Read the model definition and answer for the solid it produces. Units are mm, in the model's axes. Face numbers are marked on the shaded views. A direction names the side the tool comes from. Give positions to 0.01 mm unless a question says otherwise; leave off trailing zeros. Loops run counter-clockwise (first coordinate to the right, second up) from the corner with the lowest first, then second, coordinate; pieces in that order, holes last. Notation, with made-up numbers: (34, 2) -> (41, 2) arc R34 cw to (41, 39) -> close; hole circle Ø8 at (87.25, -16.5). An arc over 180 degrees is marked (long way). Write each question's results on one line, items separated by ' | '. Start each with the question number.
Item 1: Determine the mould class of the marked faces 3, 4 and 5 for opening direction Z: +Z half, -Z half, draft (parallel to the pull), parting line (faces both ways), or undercut.
Item 2: Find the intervals of material crossed by line 1 (Z direction, x = 0, y = -15); line 2 (Z direction, x = 0, y = -5); line 3 (Y direction, x = -19.5, z = -22), in increasing order.
Item 3: Section B-B on y = -27.5 is taken. Write down the section's boundary in (x, z), and give its area (3 significant figures).
Item 4: Which of the six approach directions +Z, -Z, +X, -X, +Y, -Y give full straight-line access (tool end or side, diameter ignored) to the marked faces 1 and 2?
Item 5: Each of these flat-tipped pins is pushed along its axis until it touches: P1, Ø10, axis at y = -14.5, z = -23.5, coming from the -X side; P2, Ø1, axis at x = 9.5, z = -22, coming from the -Y side; P3, Ø5, axis at x = -1, y = -23, coming from the -Z side. Where does it stop, or does it pass through?
Item 6: Section A-A on x = 0 is taken. Write down the section's boundary in (y, z), and give its area (3 significant figures).
Item 7: Section C-C on z = 0 is taken. Write down the section's boundary in (x, y).
Item 8: Section D-D on z = 25 is taken. Write down the section's boundary in (x, y), and give its area (3 significant figures).
```python
from build123d import *

# Parameters (mm, degrees)
F0_R     = 32.5
F1_DEPTH = 8
F2_R     = 20
F3_DEPTH = 31
F4_R     = 6
F5_DEPTH = 25
F7_DEPTH = 25.4
F8_R     = 2.25
F9_DEPTH = 8


with BuildPart() as f1:
    # F0 (on Front) → F1 (new body)
    with BuildSketch(Plane.XZ):
        Circle(F0_R)
    extrude(amount=F1_DEPTH)

    # F2 (on face) → F3 (join)
    with BuildSketch(Plane.XZ.offset(8)):
        Circle(F2_R)
    extrude(amount=F3_DEPTH)

    # F4 (on face) → F5 (cut)
    with BuildSketch(Plane.XZ.offset(39)):
        Circle(F4_R)
    extrude(amount=-F5_DEPTH, mode=Mode.SUBTRACT)

    # F6 (on face) → F7 (cut)
    with BuildSketch(Plane.XZ.offset(39)):
        Polygon((-1, 5.287178), (0, 5.287178), (1, 5.287178), (1, 7.165323), (-1, 7.165323), align=None)
    extrude(amount=-F7_DEPTH, mode=Mode.SUBTRACT)

    # F8 (on face) → F9 (cut, through all)
    with BuildSketch(Plane(origin=(0, 0, 0), x_dir=(-1, 0, 0), z_dir=(0, 1, 0))):
        with Locations((0, 25)):
            Circle(F8_R)
        with Locations((-23.776413, 7.725425)):
            Circle(F8_R)
        with Locations((-14.694631, -20.225425)):
            Circle(F8_R)
        with Locations((14.694631, -20.225425)):
            Circle(F8_R)
        with Locations((23.776413, 7.725425)):
            Circle(F8_R)
    extrude(amount=-F9_DEPTH, mode=Mode.SUBTRACT)


solid = f1.part
```
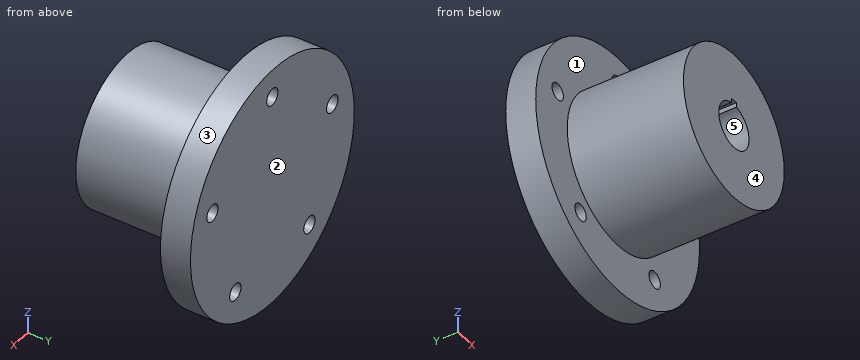
Findings:
1) face 3: parting line | face 4: draft | face 5: undercut
2) line 1: -20 to -6, 7.17 to 20 | line 2: -32.5 to 22.75, 27.25 to 32.5 | line 3: -8 to 0
3) outline: circle Ø40 at (0, 0); hole (-1, 5.92) arc R6 ccw (long way) to (1, 5.92) -> (1, 7.17) -> (-1, 7.17) -> close | area: 1,140 mm2
4) face 1: -Y | face 2: +Z, -Z, +X, -X, +Y
5) P1: x = -7.6 | P2: y = -8 | P3: z = -20
6) outline: (-39, -20) -> (-8, -20) -> (-8, -32.5) -> (0, -32.5) -> (0, 22.75) -> (-8, 22.75) -> (-8, 20) -> (-39, 20) -> (-39, 7.17) -> (-13.6, 7.17) -> (-13.6, 5.29) -> (-14, 5.29) -> (-14, -6) -> (-39, -6) -> close; (-8, 27.25) -> (0, 27.25) -> (0, 32.5) -> (-8, 32.5) -> close | area: 1,390 mm2
7) outline: (-32.5, -8) -> (-20, -8) -> (-20, -39) -> (-6, -39) -> (-6, -14) -> (6, -14) -> (6, -39) -> (20, -39) -> (20, -8) -> (32.5, -8) -> (32.5, 0) -> (-32.5, 0) -> close
8) outline: (-20.77, -8) -> (-2.25, -8) -> (-2.25, 0) -> (-20.77, 0) -> close; (2.25, -8) -> (20.77, -8) -> (20.77, 0) -> (2.25, 0) -> close | area: 296 mm2
